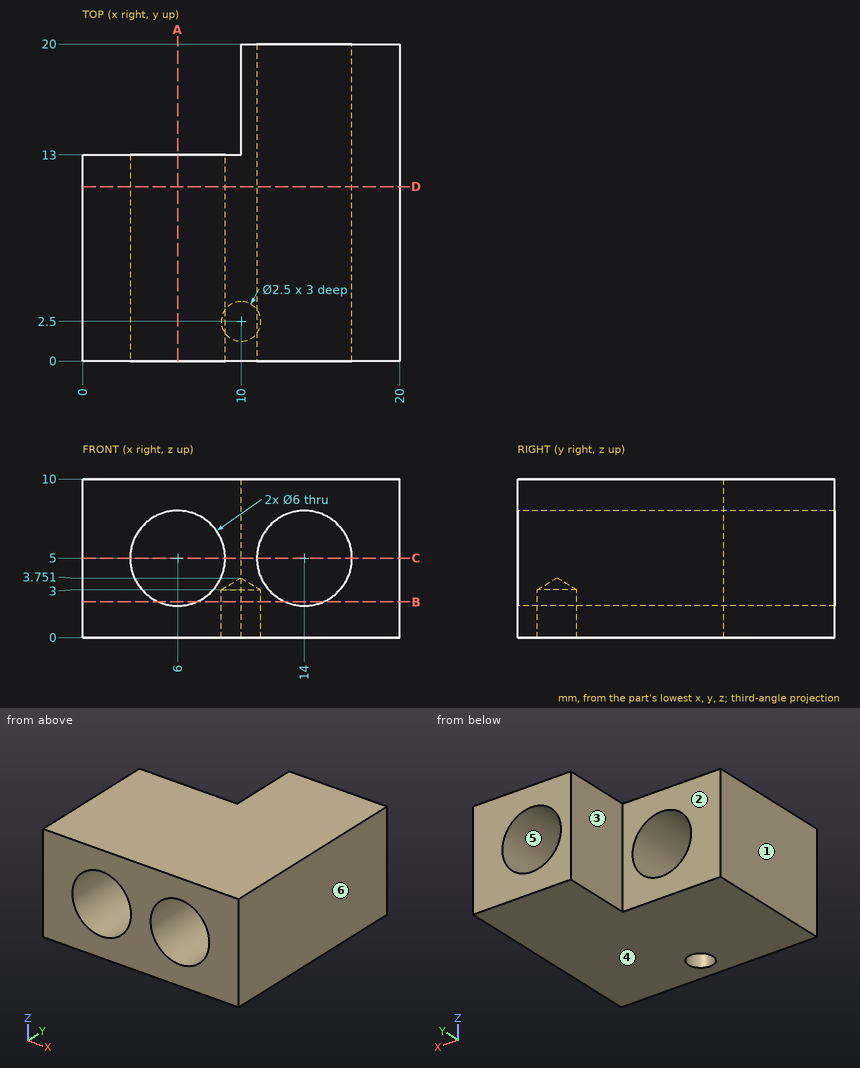
Geometry: see drawing. Coordinates: mm, zero at the bounding-box minimum. A direction names the side the tool comes from. Give positions to 0.01 mm unless a question says otherwise; leave off trailing zeros. Order: outer loops, then holes, each group sorted by start corner. A loop starts at its lowest first (then second) coordinate and runs counter-clockwise, first axis right, second up.
1. Line query: probe 1 along Z at (x, y) = (6, 8.5); probe 2 along X at (y, z) = (7.25, 2.5); probe 3 along X at (y, z) = (10.75, 5.5). Output: solid intervals per line, ascending.
Computed:
probe 1: z = 0 to 2, 8 to 10
probe 2: x = 0 to 4.34, 7.66 to 12.34, 15.66 to 20
probe 3: x = 0 to 3.04, 8.96 to 11.04, 16.96 to 20
2. Cut plane A-A (x = 6). Return loops of the section in (y, z), and give its area (3 significant figures).
Computed:
outline: (0, 0) - (13, 0) - (13, 2) - (0, 2) - close; (0, 8) - (13, 8) - (13, 10) - (0, 10) - close
area: 52.0 mm2
3. Cut plane B-B (z = 2.25). Return loops of the section in (x, y), and give its area (3 significant figures).
Computed:
outline: (0, 0) - (4.8, 0) - (4.8, 13) - (0, 13) - close; (7.2, 0) - (12.8, 0) - (12.8, 20) - (10, 20) - (10, 13) - (7.2, 13) - close; (15.2, 0) - (20, 0) - (20, 20) - (15.2, 20) - close; hole circle Ø2.5 at (10, 2.5)
area: 246 mm2
4. Draft query along X for the marked faces 3, 4, 5 and 6. Return one class per face: released by +X, released by -X, zero draft, split by the parting line, or undercut.
Computed:
face 3: released by -X
face 4: zero draft
face 5: undercut
face 6: released by +X
5. Cut plane D-D (y = 11). Return loops of the section in (x, z).
Computed:
outline: (0, 0) - (20, 0) - (20, 10) - (0, 10) - close; hole circle Ø6 at (6, 5); hole circle Ø6 at (14, 5)
6. Set-up query: the marked faces 1 and 2. Return all of +Z, -Z, +X, -X, +Y, -Y with unobstructed straight access to the full face (end or side cutting, diameter ignored); none if empty.
Computed:
face 1: +Z, -Z, -X, +Y, -Y
face 2: +Z, -Z, -X, +Y
7. Cut plane C-C (z = 5). Return loops of the section in (x, y), and give its area (3 significant figures).
Computed:
outline: (0, 0) - (3, 0) - (3, 13) - (0, 13) - close; (9, 0) - (11, 0) - (11, 20) - (10, 20) - (10, 13) - (9, 13) - close; (17, 0) - (20, 0) - (20, 20) - (17, 20) - close
area: 132 mm2
